Here's how the part is built. I have some questions about the finished solid (model axes, mm). A direction names the side the tool comes from. Give positions to 0.01 mm unless a question says otherwise; leave off trailing zeros. Write each loop counter-clockwise with the first axis right and the second up, starting at its lowest first coordinate (ties: lowest second). Pieces come first, ordered by that corner, then holes. Notation, with made-up numbers: M 15,-7.5 L 71,-7.5 A15 ccw 71,-2.5 Z; hole C -6.75,76 d5. An arc over 180 degrees is marked long. Answer as CSV lines item,"result". Start each with the question number.
Q1. If I drill on line 1 along Z through (x, y) = (-13, 1); line 2 along X through (y, z) = (1.75, 80.1); line 3 along Y through (x, z) = (-1.5, 50.5), over which ranges is the centre line in solid material (lowest first)?
Q2. Suppose I cut it at C-C (x = 6.5). Write out the boundary of the cut face in (y, z).
Q3. On a 3-axis mill with a long thin cutter (end or side, diameter ignored), from which of +Z, -Z, +X, -X, +Y, -Y can I reach the whole of each face in a straight line? I mean faces 4 (the flat face through (-8, 2, 75.1)), 5 (the flat face through (-13.51, 44.83, 48.23)). Say none if no direction works.
Q4. Suppose I cut it at B-B (z = 71). Write out the boundary of the cut face in (x, y), then the cut area to 3 significant figures.
Q5. Suppose I cut it at A-A (z = 80.1). Write out the boundary of the cut face in (x, y), then the cut area to 3 significant figures.
Q6. Thinking about a two-plate mould opening in Z: for faces 1 (the flat face through (-1, 5, 67)), 2 (the flat face through (-1.213, 21.579, 35.437)), 3 (the flat face through (-16.713, 41.044, 48.642)), which applies, +Z half, -Z half, draft (parallel to the pull), parting line (faces both ways), or undercut?
Q7. For pin 1 (3 mm diameter, centred on x = -6, z = 66, fed in from -Y); pin 2 (5.5 mm diameter, centred on x = -7, y = 3, fed in from -Z); pin 3 (6.5 mm diameter, centred on x = -13.1, z = 80.1, fed in from +Y); pin 4 (8 mm diameter, centred on x = -16.5, z = 51.5, fed in from +Y), each with a flat end and sliding along its axis, tell me the tip position at first contact or that it passes through.
Autodesk Inventor part; units mm, degrees
ref_plane "YZ Plane" through (0, 0, 0) normal (1, 0, 0) x (0, 1, 0)
ref_plane "XZ Plane" through (0, 0, 0) normal (0, 1, 0) x (-1, 0, 0)
ref_plane "XY Plane" through (0, 0, 0) normal (0, 0, 1) x (1, 0, 0)
sketch "Sketch2" plane through (0, 0, 0) normal (0, 1, 0) x (-1, 0, 0)
  circle A0 centre (13.1, 80.1) radius 2.75
  circle A1 centre (80.1, 13.1) radius 2.75 construction
  line L0 (13.1, 80.1) -> (13.1, 13.1)
  line L1 (13.1, 13.1) -> (80.1, 13.1)
  line L2 (3, 37.224) -> (37.224, 3)
  line L3 (3, 37.224) -> (51.4, 37.224) construction
  circle A2 centre (80.1, 13.1) radius 2.75
  line L4 (3.1, 112.1) -> (3.1, 79.1)
  line L5 (79.1, 3.1) -> (112.1, 3.1)
  circle A3 centre (13.1, 80.1) radius 5
  line L6 (13.1, 75.1) -> (3, 75.1)
  line L7 (3, 75.1) -> (3, 3)
  line L8 (13.1, 85.1) -> (0, 85.1)
  line L9 (0, 85.1) -> (0, 0)
  circle A4 centre (80.1, 13.1) radius 5
  line L10 (85.1, 13.1) -> (85.1, 0)
  line L11 (75.1, 13.1) -> (75.1, 3)
  line L12 (75.1, 3) -> (3, 3)
  line L13 (85.1, 0) -> (0, 0)
  line L14 (3, 37.224) -> (-4.0711, 30.1529)
  line L15 (3, 37.224) -> (13, 37.224) construction
  point P0 (0, 0)
  point P1 (0, 34.224)
  dimension "d11" = 48.4
  dimension "d12" = 45
  dimension "d13" = 10
  dimension "d14" = 10.1
  dimension "d15" = 13.1
  dimension "d16" = 3
  dimension "d17" = 10
  dimension "d18" = 13.1
  dimension "d19" = 10.1
  dimension "d20" = 10
  dimension "d21" = 135
extrude "Extrusion2" add sketch "Sketch2" along normal blind 5 contours L6 L7 L14 L9 L8 A3 | A3
sketch "Sketch4" plane through (-3, 0, 37.224) normal (-0.7071068, 0, -0.7071068) x (-0.7071068, 0, 0.7071068)
  line L0 (0, 0) -> (0, 5)
  line L1 (0, 5) -> (20.05, 39.7276)
  line L2 (0, 5) -> (40.1, 5) construction
  line L3 (8.5319, 46.3776) -> (-11.5181, 11.65)
  line L4 (-11.5181, 11.65) -> (0, 5)
  line L5 (8.5319, 46.3776) -> (20.05, 39.7276)
  line L6 (-4.2426, 0) -> (0, 0)
  line L7 (0, 0) -> (0, 5)
  line L8 (-4.2426, 5) -> (0, 5)
  line L9 (-4.2426, 0) -> (-4.2426, 5)
  line L10 (-4.2426, 5) -> (-4.2426, 7.4495)
  point P0 (-28.4426, 0)
  dimension "d33" = 300
  dimension "d34" = 40.1
  dimension "d35" = 13.3
extrude "Extrusion3" add sketch "Sketch4" against normal blind 4 contours L4 L3 L5 L1
sketch "Sketch6" plane through (0, -2.3485, 34.224) normal (-0.7071068, 0, -0.7071068) x (-0.7071068, 0, 0.7071068)
  line L0 (0, 2.3485) -> (0, 7.3485)
  circle A0 centre (0.9836, 15.0036) radius 2.6
  line L1 (3.7898, 7.6099) -> (-7.6418, 14.2099)
  circle A1 centre (6.9836, 25.3959) radius 2.6
  line L2 (0, 2.3485) -> (4.2426, 2.3485)
  line L3 (-7.2755, 13.9985) -> (4.2426, 7.3485)
  line L4 (11.0336, 32.4107) -> (-8.7344, -1.8285)
  line L5 (4.2426, 2.3485) -> (4.2426, 7.3485)
  line L6 (0, 7.3485) -> (4.2426, 7.3485)
  point P0 (-24.2, 2.3485)
  dimension "d38" = 5.2
  dimension "d39" = 5
  dimension "d40" = 12
extrude "Extrusion5" [suppressed]
fillet "Fillet1" [suppressed]
sketch "Sketch9" plane through (-0.1716, 0, 40.0524) normal (0.7071068, 0, 0.7071068) x (0.7071068, 0, -0.7071068)
  line L0 (0, 5) -> (-20.05, 39.7276)
  line L1 (-20.05, 39.7276) -> (-12.55, 26.7372)
  line L2 (-12.55, 26.7372) -> (-15.1481, 25.2372)
  line L3 (-15.1481, 25.2372) -> (-22.6481, 38.2276)
  line L4 (-22.6481, 38.2276) -> (-20.05, 39.7276)
  line L5 (-8.5319, 46.3776) -> (-20.05, 39.7276)
  line L6 (-14.2909, 43.0526) -> (11.2, -1.0989)
  line L7 (-8.5319, 46.3776) -> (-1.0319, 33.3872)
  line L8 (1.5662, 34.8872) -> (-5.9338, 47.8776)
  line L9 (-1.0319, 33.3872) -> (1.5662, 34.8872)
  line L10 (-5.9338, 47.8776) -> (-8.5319, 46.3776)
  point P0 (28.4426, 0)
  point P1 (4.6202, -0.5061)
  point P2 (4.1955, 0)
  dimension "d46" = 15
  dimension "d47" = 3
extrude "Extrusion6" [suppressed]
sketch "Sketch10" plane through (-17.1775, 39.7276, 51.4015) normal (-0.3535534, 0.8660254, 0.3535534) x (0.7071068, 0, 0.7071068)
  line L0 (0, 0) -> (0, 13.3)
  line L1 (0, 0) -> (4, 0)
  line L2 (4, 13.3) -> (4, 0)
  line L3 (0, 13.3) -> (4, 13.3)
  line L4 (-0.6, 8.15) -> (0, 8.15)
  line L5 (0, -1.85) -> (0, 5.15)
  line L6 (0, 5.15) -> (-0.6, 5.15)
  arc A0 (-0.6, 5.15) -> (-1.099, 4.6815) centre (-0.6, 4.65) ccw
  arc A1 (-1.7225, 4.2287) -> (-1.099, 4.6815) centre (-1.598, 4.713) ccw
  arc A2 (-1.7225, 9.0713) -> (-1.7225, 4.2287) centre (-1.1, 6.65) ccw
  arc A3 (-1.099, 8.6185) -> (-1.7225, 9.0713) centre (-1.598, 8.587) ccw
  arc A4 (-1.099, 8.6185) -> (-0.6, 8.15) centre (-0.6, 8.65) ccw
  line L7 (0, 0) -> (0, 13.3)
  line L8 (0.6, 5.35) -> (-0.6, 5.35)
  arc A5 (-0.6, 5.35) -> (-1.2986, 4.6941) centre (-0.6, 4.65) ccw
  arc A6 (-1.6727, 4.4224) -> (-1.2986, 4.6941) centre (-1.598, 4.713) ccw
  arc A7 (-1.6727, 8.8776) -> (-1.6727, 4.4224) centre (-1.1, 6.65) ccw
  arc A8 (-1.2986, 8.6059) -> (-1.6727, 8.8776) centre (-1.598, 8.587) ccw
  arc A9 (-1.2986, 8.6059) -> (-0.6, 7.95) centre (-0.6, 8.65) ccw
  line L9 (-0.6, 7.95) -> (0.6, 7.95)
  line L10 (0.3, -1.85) -> (0.3, 5.45)
  line L11 (0.3, 5.45) -> (-0.6, 5.45)
  arc A10 (-0.6, 5.45) -> (-1.3984, 4.7004) centre (-0.6, 4.65) ccw
  arc A11 (-1.6478, 4.5193) -> (-1.3984, 4.7004) centre (-1.598, 4.713) ccw
  arc A12 (-1.6478, 8.7807) -> (-1.6478, 4.5193) centre (-1.1, 6.65) ccw
  arc A13 (-1.3984, 8.5996) -> (-1.6478, 8.7807) centre (-1.598, 8.587) ccw
  arc A14 (-1.3984, 8.5996) -> (-0.6, 7.85) centre (-0.6, 8.65) ccw
  line L12 (-0.6, 7.85) -> (0.4, 7.85)
  line L13 (0.4, -1.85) -> (0.4, 5.55)
  line L14 (0.4, 5.55) -> (-0.6, 5.55)
  arc A15 (-0.6, 5.55) -> (-1.4982, 4.7067) centre (-0.6, 4.65) ccw
  arc A16 (-1.6229, 4.6161) -> (-1.4982, 4.7067) centre (-1.598, 4.713) ccw
  arc A17 (-1.6229, 8.6839) -> (-1.6229, 4.6161) centre (-1.1, 6.65) ccw
  arc A18 (-1.4982, 8.5933) -> (-1.6229, 8.6839) centre (-1.598, 8.587) ccw
  arc A19 (-1.4982, 8.5933) -> (-0.6, 7.75) centre (-0.6, 8.65) ccw
  line L15 (-0.6, 7.75) -> (0.4, 7.75)
  point P0 (-24.2, 22.132)
  point P1 (-11.4165, -11.1867)
  point P2 (0, 6.65)
  point P3 (0, 6.65)
  point P4 (0, 5.35)
  point P5 (0, 7.95)
  point P6 (0, 5.45)
  point P7 (0, 7.85)
  point P8 (0, 5.55)
  point P9 (0, 7.75)
  dimension "d64" = 2.5
  dimension "d65" = 0.6
  dimension "d66" = 1.1
  dimension "d67" = 0.2
  dimension "d68" = 0.3
  dimension "d69" = 0.4
extrude "Extrusion7" add sketch "Sketch10" against normal up to surface (40.1 mm away) contours L14 A15 A16 A17 A18 A19 L15 L0
sketch "Sketch11" plane through (-14.3491, 39.7276, 54.2299) normal (-0.3535534, 0.8660254, 0.3535534) x (0.7071068, 0, 0.7071068)
  line L0 (-4, 7.75) -> (-4, 13.3)
  line L1 (-4, 0) -> (0, 0)
  line L2 (0, 13.3) -> (0, 0)
  line L3 (-4, 13.3) -> (0, 13.3)
  line L4 (0, 0) -> (0, 13.3)
  line L5 (0, 0) -> (-7.3, 0)
  line L6 (-7.7, 13.3) -> (0, 13.3)
  line L7 (0, 13.3) -> (0, 0)
  line L8 (-4, 0) -> (-4, 5.55)
  line L9 (-4, 7.75) -> (-4.6, 7.75)
  arc A0 (-5.4982, 8.5933) -> (-4.6, 7.75) centre (-4.6, 8.65) ccw
  arc A1 (-5.4982, 8.5933) -> (-5.6229, 8.6839) centre (-5.598, 8.587) ccw
  arc A2 (-5.6229, 8.6839) -> (-5.6229, 4.6161) centre (-5.1, 6.65) ccw
  arc A3 (-5.6229, 4.6161) -> (-5.4982, 4.7067) centre (-5.598, 4.713) ccw
  arc A4 (-4.6, 5.55) -> (-5.4982, 4.7067) centre (-4.6, 4.65) ccw
  line L10 (-4.6, 5.55) -> (-4, 5.55)
  line L11 (-7.2, 13.3) -> (-7.2, 0)
  arc A5 (-5.6229, 8.6839) -> (-5.6229, 4.6161) centre (-5.1, 6.65) ccw
  point P0 (-28.2, 22.132)
  point P1 (-4, 0)
  point P2 (0, 13.3)
  point P3 (0, 0)
  point P4 (-4, 13.3)
  point P5 (0, 0)
  point P6 (-4, 13.3)
  point P7 (-4, 0)
  point P8 (-7.2, 6.65)
  point P9 (-7.2, 6.65)
  point P10 (-4, 0)
extrude "Extrusion8" add sketch "Sketch11" along normal blind 2
sketch "Sketch12" plane through (7.973, 11.65, 31.9078) normal (0.3535534, -0.8660254, -0.3535534) x (0.7071068, 0, 0.7071068)
  line L0 (31.9748, 40.7808) -> (-4, 9.6258)
  line L1 (-4, 0) -> (-4, 5.55)
  line L2 (-4, 0) -> (0, 0)
  line L3 (0, 13.3) -> (0, 0)
  line L4 (-4, 13.3) -> (0, 13.3)
  line L5 (-4, 7.75) -> (-4, 13.3)
  line L6 (-4.6, 7.75) -> (-4, 7.75)
  arc A0 (-5.4982, 8.5933) -> (-4.6, 7.75) centre (-4.6, 8.65) ccw
  arc A1 (-5.4982, 8.5933) -> (-5.6229, 8.6839) centre (-5.598, 8.587) ccw
  arc A2 (-5.6229, 8.6839) -> (-5.6229, 4.6161) centre (-5.1, 6.65) ccw
  arc A3 (-5.6229, 4.6161) -> (-5.4982, 4.7067) centre (-5.598, 4.713) ccw
  arc A4 (-4.6, 5.55) -> (-5.4982, 4.7067) centre (-4.6, 4.65) ccw
  line L7 (-4, 5.55) -> (-4.6, 5.55)
  point P0 (-28.2, -8.832)
extrude "Extrusion9" add sketch "Sketch12" along normal up to surface surface through (-9.05, 0, 59.662) normal (0, 1, 0)
properties part number "Pixy2 mount"
Resolved:
1,line 1,"75.1 to 77.35, 82.85 to 85.1"
1,line 2,"-18.1 to -15.85, -10.35 to 0"
1,line 3,"0 to 5"
2,outline,"M 0,27.72 L 8.33,27.72 L 11.65,30.43 L 15.26,33.38 L 0,33.38 Z"
3,face 4,"-Z, -X, +Y, -Y"
3,face 5,"+Z, -X, +Y"
4,outline,"M -3,0 L 0,0 L 0,5 L -3,5 Z"
4,area,"15.0 mm^2"
5,outline,"M -18.1,0 L -15.85,0 L -15.85,5 L -18.1,5 Z; M -10.35,0 L 0,0 L 0,5 L -10.35,5 Z"
5,area,"63.0 mm^2"
6,face 1,"draft"
6,face 2,"-Z half"
6,face 3,"undercut"
7,pin 1,"through"
7,pin 2,"z = 75.1"
7,pin 3,"y = 5"
7,pin 4,"y = 44.58"
